from build123d import *

# Parameters (mm, degrees)
SKETCH1_R           = 8
SKETCH1_R_2         = 6
BOSS_EXTRUDE1_DEPTH = 30
BOSS_EXTRUDE2_REACH = 35
SKETCH3_R           = 8
SKETCH4_R           = 6
CUT_EXTRUDE1_DEPTH  = 25


with BuildPart() as part:
    # Sketch1 → Boss-Extrude1 (new body, symmetric)
    with BuildSketch(Plane(origin=(0, 0, 0), x_dir=(0, 0, -1), z_dir=(1, 0, 0))):
        Circle(SKETCH1_R)
        Circle(SKETCH1_R_2, mode=Mode.SUBTRACT)
    extrude(amount=BOSS_EXTRUDE1_DEPTH, both=True)

    # Sketch3 → Boss-Extrude2 (add, up to next)
    with BuildSketch(Plane(origin=(0, 25, 0), x_dir=(1, 0, 0), z_dir=(0, 1, 0)), mode=Mode.PRIVATE) as boss_extrude2_sk1:
        Circle(SKETCH3_R)
    boss_extrude2_tool1 = extrude(boss_extrude2_sk1.sketch, amount=-BOSS_EXTRUDE2_REACH, mode=Mode.PRIVATE) - part.part
    add(boss_extrude2_tool1.solids().sort_by_distance((0, 25, 0))[0])

    # Sketch4 → Cut-Extrude1 (cut)
    with BuildSketch(Plane(origin=(0, 25, 0), x_dir=(1, 0, 0), z_dir=(0, 1, 0))):
        Circle(SKETCH4_R)
    extrude(amount=-CUT_EXTRUDE1_DEPTH, mode=Mode.SUBTRACT)


solid = part.part
CAD build for the part. Positions are in the model's coordinates, mm. A direction names the side the tool comes from. Give positions to 0.01 mm unless a question says otherwise; leave off trailing zeros. Loops run counter-clockwise (first coordinate to the right, second up) from the corner with the lowest first, then second, coordinate; pieces in that order, holes last. Notation, with made-up numbers: M 19,25.5 L 56,25.5 A7 ccw 56,34.5 Z; hole C 53.5,-6.5 d5. An arc over 180 degrees is marked long. Answer in a Markdown table with one row per item. Add a question column.
Item 1: Band-saw the part on A-A on z = 0. Give the cut face in (x, y).
Item 2: Band-saw the part on D-D on z = -4. Give the cut face in (x, y), then the cut area to 3 significant figures.
Item 3: Tool access for faces 5 (the face through (-1.041, 15.453, -7.932)), 6 (the face through (-30, 6, 2)): list every direction of +Z, -Z, +X, -X, +Y, -Y with a clear straight run to the whole face (end or side of a thin tool).
Item 4: Drop flat-ended pins along their axis: P1, Ø8, axis at x = -19, y = 13, coming from the +Z side; P2, Ø5, axis at x = 6.5, y = 10, coming from the -Z side; P3, Ø8, axis at x = 21.5, z = 5.5, coming from the -Y side; P4, Ø8, axis at x = 23.5, y = 7.5, coming from the -Z side. Give the stop position or say it passes through.
Item 5: Band-saw the part on B-B on y = -2.5. Give the cut face in (x, z).
Item 6: Probe probe 1 along Y at (x, z) = (10, 0); probe 2 along Y at (x, z) = (16, -1.5). List the from-to ranges inside material, lowest first.
Item 7: Band-saw the part on C-C on x = 0. Give the cut face in (y, z), then the cut area to 3 significant figures.
Item 8: Mould opens along Y. For faces 1 (the face through (-2, 25, -6)), 2 (the face through (0.42, -7.81, 1.73)), 3 (the face through (5.723, 15.453, -1.802)), 4 (the face through (-0.42, -5.857, 1.301)) say: +Y half, -Y half, draft (parallel to the pull), parting line (faces both ways), or undercut.
Reply:
| question | item | result |
|---|---|---|
| 1 | outline | M -30,-8 L 30,-8 L 30,-6 L -30,-6 Z; M -30,6 L -6,6 L -6,25 L -8,25 L -8,8 L -30,8 Z; M 6,6 L 30,6 L 30,8 L 8,8 L 8,25 L 6,25 Z |
| 2 | outline | M -30,-6.93 L 30,-6.93 L 30,-4.47 L -30,-4.47 Z; M -30,4.47 L -4.47,4.47 L -4.47,25 L -6.93,25 L -6.93,6.93 L -30,6.93 Z; M 4.47,4.47 L 30,4.47 L 30,6.93 L 6.93,6.93 L 6.93,25 L 4.47,25 Z |
| 2 | area | 362 mm^2 |
| 3 | face 5 | +Y |
| 3 | face 6 | +Z, -Z, -X, +Y, -Y |
| 4 | P1 | passes through |
| 4 | P2 | stops at z = -6.93 |
| 4 | P3 | stops at y = -7.86 |
| 4 | P4 | stops at z = -7.19 |
| 5 | outline | M -30,-7.6 L 30,-7.6 L 30,-5.45 L -30,-5.45 Z; M -30,5.45 L 30,5.45 L 30,7.6 L -30,7.6 Z |
| 6 | probe 1 | y = -8 to -6, 6 to 8 |
| 6 | probe 2 | y = -7.86 to -5.81, 5.81 to 7.86 |
| 7 | outline | M 0,-8 L 25,-8 L 25,-6 L 0,-6 A6 cw 0,6 L 25,6 L 25,8 L 0,8 A8 ccw Z |
| 7 | area | 144 mm^2 |
| 8 | face 1 | +Y half |
| 8 | face 2 | parting line |
| 8 | face 3 | draft |
| 8 | face 4 | undercut |
